Autodesk Inventor part; units mm, degrees
ref_plane "YZ Plane" through (0, 0, 0) normal (1, 0, 0) x (0, 1, 0)
ref_plane "XZ Plane" through (0, 0, 0) normal (0, 1, 0) x (-1, 0, 0)
ref_plane "XY Plane" through (0, 0, 0) normal (0, 0, 1) x (1, 0, 0)
sketch "Sketch2" plane through (0, 0, 0) normal (0, 0, 1) x (1, 0, 0)
  line L0 (-54, -101) -> (54, -101)
  line L1 (54, -101) -> (54, 101)
  line L2 (54, 101) -> (-54, 101)
  line L3 (-54, 101) -> (-54, -101)
  line L4 (-54, -101) -> (54, 101) construction
  line L5 (54, -101) -> (-54, 101) construction
  line L6 (-104, -151) -> (104, -151)
  line L7 (104, -151) -> (104, 151)
  line L8 (104, 151) -> (-104, 151)
  line L9 (-104, 151) -> (-104, -151)
  point P0 (0, 0)
  dimension "d29" = 108
  dimension "d30" = 202
  dimension "d31" = 50
extrude "Plate2" add sketch "Sketch2" along normal blind 10 contours L3 L2 L1 L0 | L9 L8 L7 L6
sketch "Sketch5" plane through (0, 0, 10) normal (0, 0, 1) x (1, 0, 0)
  line L0 (104, -151) -> (-104, -151) construction
  line L1 (104, 151) -> (104, -151) construction
  line L2 (-104, 151) -> (104, 151) construction
  line L3 (-104, -151) -> (-104, 151) construction
  line L4 (-85, 132) -> (85, 132) construction
  line L5 (85, 132) -> (85, -132) construction
  line L6 (85, -132) -> (-85, -132) construction
  line L7 (-85, -132) -> (-85, 132) construction
  circle A0 centre (-85, -132) radius 8.5
  circle A1 centre (-85, 132) radius 8.5
  circle A2 centre (-85, 0) radius 8.5
  circle A3 centre (-85, -66) radius 8.5
  circle A4 centre (-85, 64.5) radius 8.5
  line L8 (-50, -0.75) -> (50, -0.75) construction
  circle A5 centre (-31, -132) radius 8.5
  circle A6 centre (-31, -66) radius 8.5
  circle A7 centre (-31, 0) radius 8.5
  circle A8 centre (-31, 64.5) radius 8.5
  circle A9 centre (-31, 132) radius 8.5
  circle A10 centre (23, -132) radius 8.5
  circle A11 centre (23, -66) radius 8.5
  circle A12 centre (23, 0) radius 8.5
  circle A13 centre (23, 64.5) radius 8.5
  circle A14 centre (23, 132) radius 8.5
  circle A15 centre (77, -132) radius 8.5
  circle A16 centre (77, -66) radius 8.5
  circle A17 centre (77, 0) radius 8.5
  circle A18 centre (77, 64.5) radius 8.5
  circle A19 centre (77, 132) radius 8.5
  point P0 (0, 0)
  point P1 (0, -132)
  dimension "d33" = 17
  dimension "d34" = 19
  dimension "d35" = 66
  dimension "d36" = 66
  dimension "d39" = 54
extrude "Cut3" cut sketch "Sketch5" against normal blind 10 contours A0 | A1 | A2 | A3 | A4 | A5 | A9 | A10 | A14 | A15 | A16 | A17 | A18 | A19
fillet "Corner Round1" radius 6 4 edges at (-104, -151, 5) (-104, 151, 5) (104, 151, 5) (104, -151, 5)
equation "\"d35\" = d36"
equation "\"d44\" = Thickness"
equation "\"d14\" = Thickness"
equation "\"BendReliefDepth\" = 0.5 * Thickness"
equation "\"TransitionRadius\" = BendRadius"
equation "\"JacobiRadiusSize\" = BendRadius"
properties part number "PRS 1200-07 charging flange rect" material "Steel"
Work out the finished part from the listing and answer in its coordinate system (mm). Coordinates: 2 decimals unless noted, no trailing zeros. Loops run counter-clockwise (first coordinate to the right, second up) from the corner with the lowest first, then second, coordinate; pieces in that order, holes last. Notation, with made-up numbers: (43.25, -16.75) - (57.25, -16.75) arc R16 cw to (57.25, 2.25) - close; hole circle Ø5 at (54, -11). An arc over 180 degrees is marked (long way). Use a Markdown table: item, result.
Item 1: Given pin 1 Ø4 at (x, y) = (60.5, -90.5) entering from -Z; pin 2 Ø10 at (x, y) = (77, 132) entering from -Z, each flat-ended and moving along its own axis, determine where each tip first touches the part or whether it passes through.
Evaluation:
| item | result |
|---|---|
| pin 1 | stops at z = 0 |
| pin 2 | passes through |
Item 2: Find section D-D, the plane x = -31. Determine the outline of the cut face in (y, z), and give its area (3 significant figures).
Evaluation:
| item | result |
|---|---|
| outline | (-151, 0) - (-140.5, 0) - (-140.5, 10) - (-151, 10) - close; (-123.5, 0) - (123.5, 0) - (123.5, 10) - (-123.5, 10) - close; (140.5, 0) - (151, 0) - (151, 10) - (140.5, 10) - close |
| area | 2,680 mm2 |
Item 3: Consider probe 1 along Y at (x, z) = (77, 6.5); probe 2 along X at (y, z) = (-132.5, 4); probe 3 along Y at (x, z) = (22, 1). Determine where each line is inside the solid, lowest interval first. Write a range as from..to.
Evaluation:
| item | result |
|---|---|
| probe 1 | y = -151..-140.5, -123.5..-74.5, -57.5..-8.5, 8.5..56, 73..123.5, 140.5..151 |
| probe 2 | x = -104..-93.49, -76.51..-39.49, -22.51..14.51, 31.49..68.51, 85.49..104 |
| probe 3 | y = -151..-140.44, -123.56..123.56, 140.44..151 |
Item 4: Find section C-C, the plane z = 3.5. State how many separate pieces and enclosed holes the cut face has, and give its area (3 significant figures).
Evaluation:
| item | result |
|---|---|
| separate pieces | 1 |
| enclosed holes | 14 |
| area | 59,600 mm2 |
Item 5: Find section A-A, the plane x = 77. Determine the outline of the cut face in (y, z).
Evaluation:
| item | result |
|---|---|
| outline | (-151, 0) - (-140.5, 0) - (-140.5, 10) - (-151, 10) - close; (-123.5, 0) - (-74.5, 0) - (-74.5, 10) - (-123.5, 10) - close; (-57.5, 0) - (-8.5, 0) - (-8.5, 10) - (-57.5, 10) - close; (8.5, 0) - (56, 0) - (56, 10) - (8.5, 10) - close; (73, 0) - (123.5, 0) - (123.5, 10) - (73, 10) - close; (140.5, 0) - (151, 0) - (151, 10) - (140.5, 10) - close |
Item 6: Find section B-B, the plane y = 132. Determine the outline of the cut face in (x, z), and give its area (3 significant figures).
Evaluation:
| item | result |
|---|---|
| outline | (-104, 0) - (-93.5, 0) - (-93.5, 10) - (-104, 10) - close; (-76.5, 0) - (-39.5, 0) - (-39.5, 10) - (-76.5, 10) - close; (-22.5, 0) - (14.5, 0) - (14.5, 10) - (-22.5, 10) - close; (31.5, 0) - (68.5, 0) - (68.5, 10) - (31.5, 10) - close; (85.5, 0) - (104, 0) - (104, 10) - (85.5, 10) - close |
| area | 1,400 mm2 |
Item 7: The mould has two halves that part along Y. Classify faces 1 (the flat face through (-1, -151, 5)), 2 (the flat face through (-1, 2, 0)), 3 (the cylindrical face through (21.16, 123.7, 5.07)): +Y half, -Y half, draft (parallel to the pull), parting line (faces both ways), or undercut.
Evaluation:
| item | result |
|---|---|
| face 1 | -Y half |
| face 2 | draft |
| face 3 | undercut |
